For this review, take the finished solid that the model builds, in its own axes (mm). Face numbers are marked on the shaded views. A direction names the side the tool comes from. Give positions to 0.01 mm unless a question says otherwise; leave off trailing zeros. Use CSV: the item, a comma, the result in double quotes. Start each with the question number.
1. Tool access review of the marked faces 4, 5 and 6: name each direction out of +Z, -Z, +X, -X, +Y, -Y from which nothing blocks a thin tool from reaching the whole face with its end or side.
2. The part is to be moulded in two halves that separate along Y. For the marked faces 1, 2 and 3, say which applies: pulls with the +Y half, pulls with the -Y half, needs draft (parallel to the pull), parting line crosses it, or undercut.
3. Take a section at D-D, the plane z = -2.5. State how many separate pieces and enclosed holes the cut face has, and give its area (3 significant figures).
4. To check wall thickness, follow line 1 (X direction, y = -5.5, z = -3) (3 decimals); line 2 (X direction, y = -1, z = -4). State the ranges of each line that lie inside material, in increasing order. Write a range as [from, to].
5. Insertion check: P1, Ø5, axis at x = 4, y = -1, coming from the +Z side; P2, Ø5, axis at x = 1.5, z = -7, coming from the -Y side; P3, Ø5, axis at y = 2, z = -10.5, coming from the +X side; P4, Ø3, axis at y = 1, z = -5, coming from the -X side. Each pin has a flat end and moves straight along its axis. Give the tip position at first contact, or say it passes through.
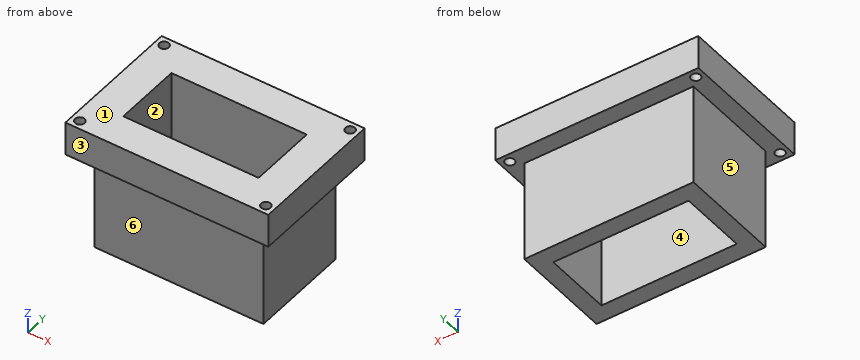
from build123d import *

# Parameters (mm, degrees)
F1_DEPTH = 3.175
F2_DEPTH = 12.7
F3_R     = 0.4445
F4_DEPTH = 25.4


with BuildPart() as f1:
    # F0 (on Top) → F1 (new body)
    with BuildSketch(Plane.XY):
        Polygon((-7.9375, 4.7625), (0, 4.7625), (0, 6.35), (-9.525, 6.35), (-9.525, -6.35), (-7.9375, -4.7625), align=None)
        Polygon((0, 6.35), (0, 4.7625), (7.9375, 4.7625), (7.9375, -4.7625), (0, -4.7625), (0, -6.35), (9.525, -6.35), (9.525, 6.35), align=None)
        Polygon((0, -6.35), (0, -4.7625), (-7.9375, -4.7625), (-9.525, -6.35), align=None)
        Polygon((0, -4.7625), (0, -3.175), (-6.35, -3.175), (-7.9375, -4.7625), align=None)
        Polygon((-6.35, 3.175), (0, 3.175), (0, 4.7625), (-7.9375, 4.7625), (-7.9375, -4.7625), (-6.35, -3.175), align=None)
        Polygon((0, 3.175), (6.35, 3.175), (6.35, -3.175), (0, -3.175), (0, -4.7625), (7.9375, -4.7625), (7.9375, 4.7625), (0, 4.7625), align=None)
    extrude(amount=-F1_DEPTH)

    # F0 (on Top) → F2 (join)
    with BuildSketch(Plane.XY):
        Polygon((0, -4.7625), (0, -3.175), (-6.35, -3.175), (-7.9375, -4.7625), align=None)
        Polygon((0, 3.175), (6.35, 3.175), (6.35, -3.175), (0, -3.175), (0, -4.7625), (7.9375, -4.7625), (7.9375, 4.7625), (0, 4.7625), align=None)
        Polygon((-6.35, 3.175), (0, 3.175), (0, 4.7625), (-7.9375, 4.7625), (-7.9375, -4.7625), (-6.35, -3.175), align=None)
    extrude(amount=-F2_DEPTH)

    # F3 (on face) → F4 (cut)
    with BuildSketch(Plane(origin=(0, 0, -3.175), x_dir=(1, 0, 0), z_dir=(0, 0, -1))):
        with Locations((-8.73125, 5.55625)):
            Circle(F3_R)
        with Locations((8.73125, 5.55625)):
            Circle(F3_R)
        with Locations((8.73125, -5.55625)):
            Circle(F3_R)
        with Locations((-8.73125, -5.55625)):
            Circle(F3_R)
    extrude(amount=-F4_DEPTH, mode=Mode.SUBTRACT)


solid = f1.part
Result set:
1,face 4,"+Z, -Z"
1,face 5,"-Z, -X, +Y, -Y"
1,face 6,"-Z, +X, -X, -Y"
2,face 1,"needs draft"
2,face 2,"undercut"
2,face 3,"pulls with the -Y half"
3,separate pieces,"1"
3,enclosed holes,"5"
3,area,"159 mm2"
4,line 1,"[-9.525, -9.172], [-8.29, 8.29], [9.172, 9.525]"
4,line 2,"[-7.94, -6.35], [6.35, 7.94]"
5,P1,"z = 0"
5,P2,"y = -4.76"
5,P3,"x = 7.94"
5,P4,"x = -7.94"
